Build history of the part. All positions in model axes, mm. Face numbers are marked on the shaded views. A direction names the side the tool comes from. Give positions to 0.01 mm unless a question says otherwise; leave off trailing zeros. Loops run counter-clockwise (first coordinate to the right, second up) from the corner with the lowest first, then second, coordinate; pieces in that order, holes last.
1) Band-saw the part on A-A on y = 199. List the corners of the cut face in (x, z).
2) Two-plate mould, pull along Y, no slides. Class the marked faces 1, 2 and 3: +Y half, -Y half, draft (parallel to the pull), parting line (faces both ways), or undercut.
3) Band-saw the part on C-C on y = 50.8. List the corners of the cut face in (x, z).
4) Band-saw the part on B-B on x = 488.95. List the corners of the cut face in (y, z), then the cut area to 3 significant figures.
5) Wall check: line 1 (X direction, y = 50, z = 238); line 2 (X direction, y = 181.5, z = 42.5); line 3 (Y direction, x = 488.95, z = 239.75). Give the ranges that are in metal, low to high.
6) 3-axis set-ups, long thin cutter, end or side, ignore diameter. For the marked faces 4 and 5: which of +Z, -Z, +X, -X, +Y, -Y reach the whole face in a straight line?
7) Band-saw the part on D-D on z = 95. List the corners of the cut face in (x, y).
Autodesk Inventor part; units mm, degrees
ref_plane "YZ Plane" through (0, 0, 0) normal (1, 0, 0) x (0, 1, 0)
ref_plane "XZ Plane" through (0, 0, 0) normal (0, 1, 0) x (-1, 0, 0)
ref_plane "XY Plane" through (0, 0, 0) normal (0, 0, 1) x (1, 0, 0)
sketch "Sketch1" plane through (0, 0, 0) normal (0, 0, 1) x (1, 0, 0)
  line L0 (0, 0) -> (584.2, 0)
  line L1 (584.2, 0) -> (584.2, 431.8)
  line L2 (584.2, 431.8) -> (0, 431.8)
  line L3 (0, 431.8) -> (0, 0)
  line L4 (6.35, 6.35) -> (577.85, 6.35)
  line L5 (577.85, 6.35) -> (577.85, 425.45)
  line L6 (577.85, 425.45) -> (6.35, 425.45)
  line L7 (6.35, 425.45) -> (6.35, 6.35)
  dimension "d0" = 6.35
  dimension "d1" = 6.35
  dimension "d2" = 6.35
  dimension "d3" = 6.35
  dimension "d4" = 584.2
  dimension "d5" = 431.8
extrude "Extrusion1" add sketch "Sketch1" along normal blind 241.3
sketch "Sketch2" plane through (6.35, 6.35, 241.3) normal (1, 0, 0) x (0, 0, -1)
  line L0 (0, 0) -> (0, 419.1)
  line L1 (241.3, 0) -> (0, 0)
  line L2 (0, 419.1) -> (6.35, 419.1)
  line L3 (6.35, 419.1) -> (6.35, 0)
  line L4 (6.35, 0) -> (0, 0)
  line L5 (0, 0) -> (0, 419.1)
  point P0 (241.3, -6.35)
  dimension "d8" = 6.35
extrude "Extrusion2" add sketch "Sketch2" along normal blind 152.4
sketch "Sketch3" plane through (577.85, 6.35, 241.3) normal (-1, 0, 0) x (0, 0, 1)
  line L0 (0, 419.1) -> (0, 0)
  line L1 (-241.3, 419.1) -> (0, 419.1)
  line L2 (0, 0) -> (-6.35, 0)
  line L3 (-6.35, 0) -> (-6.35, 419.1)
  line L4 (-6.35, 419.1) -> (0, 419.1)
  line L5 (0, 419.1) -> (0, 0)
  point P0 (-241.3, -6.35)
  dimension "d11" = 6.35
extrude "Extrusion3" add sketch "Sketch3" along normal blind 152.4
sketch "Sketch4" plane through (0, 0, 241.3) normal (0, 0, 1) x (1, 0, 0)
  line L0 (57.15, 381) -> (76.2, 381)
  line L1 (76.2, 381) -> (76.2, 342.9)
  line L2 (76.2, 342.9) -> (57.15, 342.9)
  line L3 (57.15, 342.9) -> (57.15, 381)
  line L4 (0, 0) -> (0, 431.8)
  line L5 (0, 431.8) -> (584.2, 431.8)
  dimension "d14" = 19.05
  dimension "d15" = 38.1
  dimension "d29" = 57.15
  dimension "d30" = 50.8
extrude "Extrusion4" cut sketch "Sketch4" against normal up to next
pattern_linear "Rectangular Pattern1" count 5 spacing 63.5 along (0, -1, 0) count 2 spacing 457.2 along (1, 0, 0) of "Extrusion4"
sketch "Sketch5" plane through (0, 0, 241.3) normal (0, 0, 1) x (1, 0, 0)
  line L0 (425.45, 425.45) -> (425.45, 6.35)
  line L1 (584.2, 0) -> (0, 0)
  circle A0 centre (488.95, 50.8) radius 12.7
  dimension "d24" = 25.4
  dimension "d25" = 63.5
  dimension "d26" = 50.8
extrude "Extrusion5" cut sketch "Sketch5" against normal up to next
properties part number "Board_Final_Concept" material "Wood (Birch)"
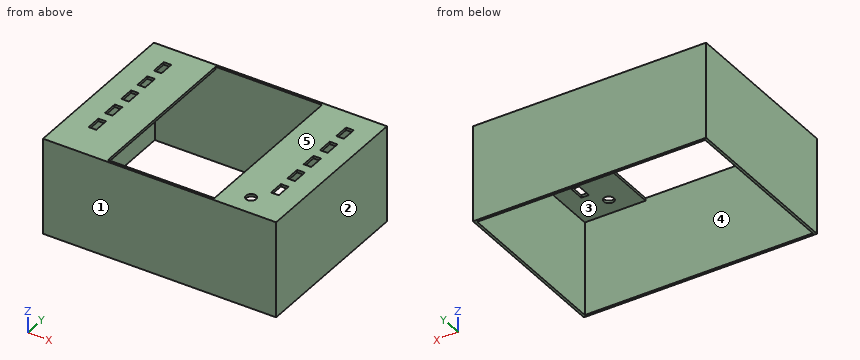
Findings below:
1. outline: (0, 0) - (6.35, 0) - (6.35, 234.95) - (158.75, 234.95) - (158.75, 241.3) - (0, 241.3) - close; (425.45, 234.95) - (577.85, 234.95) - (577.85, 0) - (584.2, 0) - (584.2, 241.3) - (425.45, 241.3) - close
2. face 1: -Y half
2. face 2: draft
2. face 3: undercut
3. outline: (0, 0) - (6.35, 0) - (6.35, 234.95) - (158.75, 234.95) - (158.75, 241.3) - (0, 241.3) - close; (425.45, 234.95) - (476.25, 234.95) - (476.25, 241.3) - (425.45, 241.3) - close; (501.65, 234.95) - (577.85, 234.95) - (577.85, 0) - (584.2, 0) - (584.2, 241.3) - (501.65, 241.3) - close
4. outline: (0, 0) - (6.35, 0) - (6.35, 234.95) - (38.1, 234.95) - (38.1, 241.3) - (0, 241.3) - close; (63.5, 234.95) - (425.45, 234.95) - (425.45, 0) - (431.8, 0) - (431.8, 241.3) - (63.5, 241.3) - close
4. area: 5,560 mm2
5. line 1: x = 0 to 158.75, 425.45 to 476.28, 501.62 to 584.2
5. line 2: x = 0 to 6.35, 577.85 to 584.2
5. line 3: y = 0 to 38.1, 63.5 to 431.8
6. face 4: -Z
6. face 5: +Z, +X, -X, +Y, -Y
7. outline: (0, 0) - (584.2, 0) - (584.2, 431.8) - (0, 431.8) - close; hole (6.35, 6.35) - (577.85, 6.35) - (577.85, 425.45) - (6.35, 425.45) - close
